from build123d import *

# Parameters (mm, degrees)
SKETCH1_R           = 20
SKETCH1_R_2         = 7.5
BOSS_EXTRUDE1_DEPTH = 15
CUT_EXTRUDE1_START  = -10
CUT_EXTRUDE1_DEPTH  = 10
SKETCH4_R           = 1.5
BOSS_EXTRUDE2_DEPTH = 10
CIRPATTERN1_COUNT   = 4


with BuildPart() as part:
    # Sketch1 → Boss-Extrude1 (new body)
    with BuildSketch(Plane(origin=(0, 0, 0), x_dir=(1, 0, 0), z_dir=(0, 1, 0))):
        with Locations(Location((0, 0, 0), (0, 0, 270))):
            Circle(SKETCH1_R)
        with Locations(Location((0, 0, 0), (0, 0, 270))):
            Circle(SKETCH1_R_2, mode=Mode.SUBTRACT)
    extrude(amount=BOSS_EXTRUDE1_DEPTH)

    # Sketch2 → Cut-Extrude1 (cut)
    with BuildSketch(Plane(origin=(0, 15, 0), x_dir=(1, 0, 0), z_dir=(0, 1, 0)).offset(CUT_EXTRUDE1_START)):
        with BuildLine():
            Line((-19.595917942, -4), (-11.842719282, -4))
            ThreePointArc((-11.842719282, -4), (-12.5, 0), (-11.842719282, 4))
            Line((-11.842719282, 4), (-19.595917942, 4))
            ThreePointArc((-19.595917942, 4), (-20, 0), (-19.595917942, -4))
        make_face()
        with BuildLine():
            Line((-4, 19.595917942), (-4, 11.842719282))
            ThreePointArc((-4, 11.842719282), (0, 12.5), (4, 11.842719282))
            Line((4, 11.842719282), (4, 19.595917942))
            ThreePointArc((4, 19.595917942), (0, 20), (-4, 19.595917942))
        make_face()
        with BuildLine():
            Line((11.842719282, 4), (19.595917942, 4))
            ThreePointArc((19.595917942, 4), (20, 0), (19.595917942, -4))
            Line((19.595917942, -4), (11.842719282, -4))
            ThreePointArc((11.842719282, -4), (12.5, 0), (11.842719282, 4))
        make_face()
        with BuildLine():
            Line((4, -11.842719282), (4, -19.595917942))
            ThreePointArc((4, -19.595917942), (0, -20), (-4, -19.595917942))
            Line((-4, -19.595917942), (-4, -11.842719282))
            ThreePointArc((-4, -11.842719282), (0, -12.5), (4, -11.842719282))
        make_face()
    extrude(amount=CUT_EXTRUDE1_DEPTH, mode=Mode.SUBTRACT)

    # Sketch4 → Boss-Extrude2 (add)
    with BuildSketch(Plane(origin=(0, 0, 4), x_dir=(-1, 0, 0), z_dir=(0, 0, -1))):
        with Locations(Location((-17.095917942, 10, 0), (0, 0, 180))):
            Circle(SKETCH4_R)
    boss_extrude2 = extrude(amount=BOSS_EXTRUDE2_DEPTH)

    # CirPattern1: Boss-Extrude2 ×4 about axis
    cirpattern1_axis = Axis((0, 15, 0), (0, -1, 0))
    for i in range(1, CIRPATTERN1_COUNT):
        add(boss_extrude2.rotate(cirpattern1_axis, i * 360 / CIRPATTERN1_COUNT))


solid = part.part
Read the model definition and answer for the solid it produces. Units are mm, in the model's axes. A direction names the side the tool comes from. Give positions to 0.01 mm unless a question says otherwise; leave off trailing zeros. Loops run counter-clockwise (first coordinate to the right, second up) from the corner with the lowest first, then second, coordinate; pieces in that order, holes last. Notation, with made-up numbers: (49.25, 21.5) -> (79.25, 21.5) arc R33 cw to (79.25, 56.5) -> close; hole circle Ø2 at (68.25, 15). An arc over 180 degrees is marked (long way). Use a Markdown table: item, result.
Q1. Section C-C, the plane x = 0 is taken. Determine the outline of the cut face in (y, z), then the cut area to 3 significant figures.
Solved:
| item | result |
|---|---|
| outline | (0, -20) -> (5, -20) -> (5, -12.5) -> (15, -12.5) -> (15, -7.5) -> (0, -7.5) -> close; (0, 7.5) -> (15, 7.5) -> (15, 12.5) -> (5, 12.5) -> (5, 20) -> (0, 20) -> close; circle Ø3 at (10, -17.1); circle Ø3 at (10, 17.1) |
| area | 239 mm^2 |
Q2. Each of these flat-tipped pins is pushed along its axis until it touches: pin 1 (8.5 mm diameter, centred on y = 12, z = -15.5, fed in from +X); pin 2 (2.5 mm diameter, centred on x = 0, z = -16.5, fed in from +Y); pin 3 (5 mm diameter, centred on y = 10, z = 13.5, fed in from +X). Where does it stop, or does it pass through?
Solved:
| item | result |
|---|---|
| pin 1 | stops at x = 16.54 |
| pin 2 | stops at y = 11.5 |
| pin 3 | stops at x = 16.7 |
Q3. Section A-A, the plane z = 0 is taken. Determine the outline of the cut face in (x, y), then the cut area to 3 significant figures.
Solved:
| item | result |
|---|---|
| outline | (-20, 0) -> (-7.5, 0) -> (-7.5, 15) -> (-12.5, 15) -> (-12.5, 5) -> (-20, 5) -> close; circle Ø3 at (-17.1, 10); (7.5, 0) -> (20, 0) -> (20, 5) -> (12.5, 5) -> (12.5, 15) -> (7.5, 15) -> close; circle Ø3 at (17.1, 10) |
| area | 239 mm^2 |
Q4. Determine the mould class of faces 1 (the face through (-7.66, 7.395, 18.475)), 2 (the face through (12.5, 9.9, 0.1)), 3 (the face through (0, 5, -16)) for opening direction Z: pulls with the +Z half, pulls with the -Z half, needs draft (parallel to the pull), parting line crosses it, or undercut.
Solved:
| item | result |
|---|---|
| face 1 | parting line crosses it |
| face 2 | undercut |
| face 3 | needs draft |
Q5. Find the intervals of material crossed by line 1 along X through (y, z) = (11.75, 0); line 2 along X through (y, z) = (4, 0); line 3 along Z through (x, y) = (-17.5, 8), in increasing order.
Solved:
| item | result |
|---|---|
| line 1 | x = -12.5 to -7.5, 7.5 to 12.5 |
| line 2 | x = -20 to -7.5, 7.5 to 20 |
| line 3 | z = -9.68 to -4, 4 to 9.68 |
Q6. Section D-D, the plane z = 6 is taken. Determine the outline of the cut face in (x, y).
Solved:
| item | result |
|---|---|
| outline | (-19.08, 0) -> (-4.5, 0) -> (-4.5, 15) -> (-19.08, 15) -> close; (4.5, 0) -> (19.08, 0) -> (19.08, 15) -> (4.5, 15) -> close |
Q7. A tool of negligible diameter and unlimited length cuts with its end or side. For faces 4 (the face through (-15, 10, -4)), 5 (the face through (16, 5, 0)), 6 (the face through (-16, 5, 0)), 7 (the face through (0.33, 7.395, -7.493)), 8 (the face through (0, 5, 16)), from which of +Z, -Z, +X, -X, +Y, -Y can it reach the whole face along a straight path? Write none if from no direction.
Solved:
| item | result |
|---|---|
| face 4 | none |
| face 5 | +X |
| face 6 | -X |
| face 7 | +Y, -Y |
| face 8 | +Z |
Q8. Section B-B, the plane y = 13.5 is taken. Determine the outline of the cut face in (x, z), then the cut area to 3 significant figures.
Solved:
| item | result |
|---|---|
| outline | (-19.6, -4) arc R20 ccw to (-4, -19.6) -> (-4, -11.84) arc R12.5 ccw to (4, -11.84) -> (4, -19.6) arc R20 ccw to (19.6, -4) -> (11.84, -4) arc R12.5 ccw to (11.84, 4) -> (19.6, 4) arc R20 ccw to (4, 19.6) -> (4, 11.84) arc R12.5 ccw to (-4, 11.84) -> (-4, 19.6) arc R20 ccw to (-19.6, 4) -> (-11.84, 4) arc R12.5 ccw to (-11.84, -4) -> close; hole circle Ø15 at (0, 0) |
| area | 837 mm^2 |
